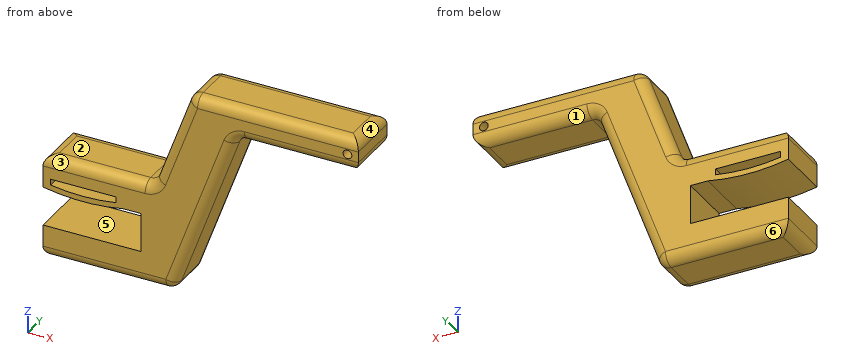
from build123d import *

# Parameters (mm, degrees)
F1_DEPTH = 25
F2_F1_R  = 5
F2_F2_R  = 5
F3_R     = 2
F4_DEPTH = 25


with BuildPart() as f1:
    # F0 (on Front) → F1 (new body)
    with BuildSketch(Plane.XZ):
        with BuildLine():
            Line((45, 15), (0, 15))
            Line((0, 15), (0, 0))
            Line((0, 0), (60, 0))
            Line((60, 0), (89.1176187413, 80))
            Line((89.1176187413, 80), (145, 80))
            Line((145, 80), (145, 95))
            Line((145, 95), (67.5712870168, 95))
            Line((67.5712870168, 95), (50.4646860063, 48))
            Line((50.4646860063, 48), (0, 48))
            Line((0, 48), (0, 33))
            ThreePointArc((0, 33), (18.5, 31.181274943), (37, 33))
            Line((37, 33), (45, 33))
            Line((45, 33), (45, 15))
        make_face()
        with BuildLine():
            ThreePointArc((33.5, 34.9055936253), (18.5, 33.681274943), (3.5, 34.9055936253))
            Line((3.5, 34.9055936253), (3.5, 37.681274943))
            Line((3.5, 37.681274943), (33.5, 37.681274943))
            Line((33.5, 37.681274943), (33.5, 34.9055936253))
        make_face(mode=Mode.SUBTRACT)
    extrude(amount=F1_DEPTH)

    # F2: fillet of radius 5 on 16 edges, made by hand

    # F2_f1
    f2_f1_edges = [f1.edges().sort_by_distance(p)[0] for p in [
        (89.1176187413, -12.5, 80),
        (50.4646860063, -12.5, 48),
    ]]
    fillet(f2_f1_edges, radius=F2_F1_R)

    # F2_f2
    f2_f2_edges = [f1.edges().sort_by_distance(p)[0] for p in [
        (60, -12.5, 0),
        (67.5712870168, -12.5, 95),
        (145, -12.5, 95),
        (145, -12.5, 80),
        (0, -12.5, 48),
        (0, -12.5, 0),
        (118.8093282162, -25, 80),
        (73.9600966642, 0, 38.3550503583),
        (106.2856435084, -25, 95),
        (59.616699218, -25, 73.1449496417),
        (106.2856435084, 0, 95),
        (59.616699218, 0, 73.1449496417),
        (30, -25, 0),
        (30, 0, 0),
        (49.831530497, 0, 48.9042397786),
        (49.831530497, -25, 48.9042397786),
        (89.7507742506, 0, 79.0957602214),
        (89.7507742506, -25, 79.0957602214),
    ]]
    fillet(f2_f2_edges, radius=F2_F2_R)

    # F3 (on face) → F4 (cut)
    with BuildSketch(Plane.XZ.offset(25)):
        with Locations((140, 87.5)):
            Circle(F3_R)
    extrude(amount=-F4_DEPTH, mode=Mode.SUBTRACT)


solid = f1.part
Work out the finished part from the listing and answer in its coordinate system (mm). Face numbers are marked on the shaded views. A direction names the side the tool comes from. Coordinates: 2 decimals unless noted, no trailing zeros. Loops run counter-clockwise (first coordinate to the right, second up) from the corner with the lowest first, then second, coordinate; pieces in that order, holes last. Notation, with made-up numbers: (-2, 71.25) -> (16, 71.25) arc R21 ccw to (16, 110.25) -> close; hole circle Ø6 at (25.5, 36.5). An arc over 180 degrees is marked (long way). Answer as CSV lines item,"result".
1) The part is cut by section A-A (y = -11). Give the vertices of the cut face in (x, z), and give its area (3 significant figures).
A:
outline,"(0, 5) arc R5 ccw to (5, 0) -> (56.5, 0) arc R5 ccw to (61.2, 3.29) -> (87.92, 76.71) arc R5 cw to (92.62, 80) -> (140, 80) arc R5 ccw to (145, 85) -> (145, 90) arc R5 ccw to (140, 95) -> (71.07, 95) arc R5 ccw to (66.37, 91.71) -> (51.66, 51.29) arc R5 cw to (46.96, 48) -> (5, 48) arc R5 ccw to (0, 43) -> (0, 33) arc R95 ccw to (37, 33) -> (45, 33) -> (45, 15) -> (0, 15) -> close; hole (3.5, 34.91) arc R92.5 ccw to (33.5, 34.91) -> (33.5, 37.68) -> (3.5, 37.68) -> close; hole circle Ø4 at (140, 87.5)"
area,"4,460 mm²"
2) Straight lines are drawn through the part: probe 1 along Z at (x, y) = (140, -5.5); probe 2 along Z at (x, y) = (111, -16.5); probe 3 along X at (y, z) = (-12, 86.5). For each, find the intervals that lie inside material, in ascending order.
A:
probe 1,"z = 80 to 85.5, 89.5 to 95"
probe 2,"z = 80 to 95"
probe 3,"x = 64.48 to 138.27, 141.73 to 145"
3) Flat-ended cylindrical pins translate along their axes: pin 1 (12 mm diameter, centred on y = -5.5, z = 17, fed in from +X); pin 2 (12.5 mm diameter, centred on x = 22, y = -7, fed in from +Z); pin 3 (4.5 mm diameter, centred on x = 140, z = 87.5, fed in from -Y); pin 4 (0.8 mm diameter, centred on y = -7.5, z = 36, fed in from +X). Find the tip coordinate at first contact, or state that the pin passes through.
A:
pin 1,"stops at x = 68.37"
pin 2,"stops at z = 48"
pin 3,"stops at y = -25"
pin 4,"stops at x = 73.25"
4) The part is cut by section C-C (x = 15.5). Give the vertices of the cut face in (y, z).
A:
outline,"(-25, 5) arc R5 ccw to (-20, 0) -> (-5, 0) arc R5 ccw to (0, 5) -> (0, 15) -> (-25, 15) -> close; (-25, 31.23) -> (0, 31.23) -> (0, 33.73) -> (-25, 33.73) -> close; (-25, 37.68) -> (0, 37.68) -> (0, 43) arc R5 ccw to (-5, 48) -> (-20, 48) arc R5 ccw to (-25, 43) -> close"
5) For the marked faces 1, 2 and 3, determine the directions among +Z, -Z, +X, -X, +Y, -Y from which every point of the face is accessible in a straight line to the end or side of a thin tool.
A:
face 1,"-Z, +X, +Y"
face 2,"+Z, -X, +Y, -Y"
face 3,"+Z, -X, -Y"
6) For a pull along Z with two mould halves and no side action, classify the marked faces 4, 5 and 6 as released by +Z, released by -Z, zero draft, split by the parting line, or undercut.
A:
face 4,"released by +Z"
face 5,"undercut"
face 6,"released by -Z"
7) The part is cut by section B-B (x = 117.5). Give the vertices of the cut face in (y, z), and give its area (3 significant figures).
A:
outline,"(-25, 85) arc R5 ccw to (-20, 80) -> (-5, 80) arc R5 ccw to (0, 85) -> (0, 90) arc R5 ccw to (-5, 95) -> (-20, 95) arc R5 ccw to (-25, 90) -> close"
area,"354 mm²"
